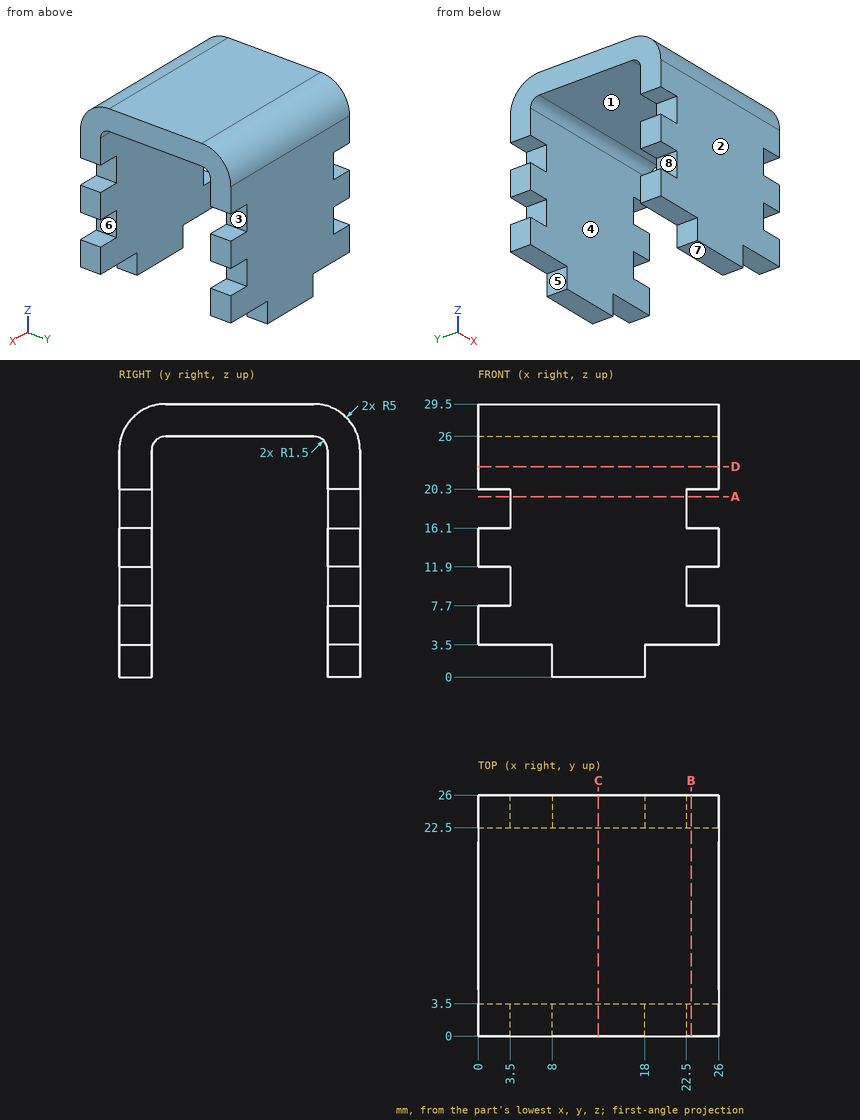
Design review of the part shown in the three views and the two pictorial views. Dimensions are in mm from the part's minimum x, y and z. A direction names the side the tool comes from. Round coordinates to 2 decimals unless told otherwise and drop trailing zeros. Write each loop counter-clockwise with the first axis right and the second up, starting at its lowest first coordinate (ties: lowest second). Pieces come first, ordered by that corner, then holes. Notation, with made-up numbers: (33.5, -5.75) -> (67.5, -5.75) arc R28 ccw to (67.5, 30.25) -> close; hole circle Ø4 at (70.5, 21). An arc over 180 degrees is marked (long way). Write item = value, one per line. Start each with the question number.
1) Take a section at B-B, the plane x = 23. State the section outline as (y, z) points, plus the area to 3 significant figures.
2) Take a section at D-D, the plane z = 22.75. State the section outline as (x, y) points.
3) Clearance check with flat-ended pins moving along their axes: pin 1 (3 mm diameter, centred on x = 1, y = 2.5, fed in from -Z); pin 2 (1 mm diameter, centred on x = 2.5, y = 1.5, fed in from +Z); pin 3 (4 mm diameter, centred on x = 23.5, y = 25, fed in from +Z). State where each tip first meets the part, or that it passes through.
4) Mouldability with a two-part tool opening along Y and no side actions: class the marked faces 1, 2 and 3 as +Y half, -Y half, draft (parallel to the pull), parting line (faces both ways), or undercut.
5) Take a section at A-A, the plane z = 19.5. State the section outline as (x, y) points.
6) Wall thickness on probe 1 along Y at (x, z) = (2, 13.25); probe 2 along Z at (x, y) = (10, 20.25); probe 3 along X at (y, z) = (22.75, 20): over which ranges is each line inside the solid? List them lowest first. Write a range as from..to.
7) Tool access review of the marked faces 4, 5, 6, 7 and 8: name each direction out of +Z, -Z, +X, -X, +Y, -Y from which nothing blocks a thin tool from reaching the whole face with its end or side.
8) Take a section at C-C, the plane x = 13. State the section outline as (y, z) points.
Results list:
q1.outline = (0, 3.5) -> (3.5, 3.5) -> (3.5, 7.7) -> (0, 7.7) -> close; (0, 11.9) -> (3.5, 11.9) -> (3.5, 16.1) -> (0, 16.1) -> close; (0, 20.3) -> (3.5, 20.3) -> (3.5, 24.5) arc R1.5 cw to (5, 26) -> (21, 26) arc R1.5 cw to (22.5, 24.5) -> (22.5, 20.3) -> (26, 20.3) -> (26, 24.5) arc R5 ccw to (21, 29.5) -> (5, 29.5) arc R5 ccw to (0, 24.5) -> close; (22.5, 3.5) -> (26, 3.5) -> (26, 7.7) -> (22.5, 7.7) -> close; (22.5, 11.9) -> (26, 11.9) -> (26, 16.1) -> (22.5, 16.1) -> close
q1.area = 180 mm²
q2.outline = (0, 0) -> (26, 0) -> (26, 3.5) -> (0, 3.5) -> close; (0, 22.5) -> (26, 22.5) -> (26, 26) -> (0, 26) -> close
q3.pin_1 = 3.5
q3.pin_2 = 28.5
q3.pin_3 = 29.08
q4.face_1 = undercut
q4.face_2 = -Y half
q4.face_3 = draft
q5.outline = (3.5, 0) -> (22.5, 0) -> (22.5, 3.5) -> (3.5, 3.5) -> close; (3.5, 22.5) -> (22.5, 22.5) -> (22.5, 26) -> (3.5, 26) -> close
q6.probe_1 = 0..3.5, 22.5..26
q6.probe_2 = 26..29.5
q6.probe_3 = 3.5..22.5
q7.face_4 = -Z, +X, -X
q7.face_5 = -Z, -X, +Y, -Y
q7.face_6 = +X, +Y, -Y
q7.face_7 = -Z, +X, -X, +Y, -Y
q7.face_8 = -X, +Y, -Y
q8.outline = (0, 0) -> (3.5, 0) -> (3.5, 24.5) arc R1.5 cw to (5, 26) -> (21, 26) arc R1.5 cw to (22.5, 24.5) -> (22.5, 0) -> (26, 0) -> (26, 24.5) arc R5 ccw to (21, 29.5) -> (5, 29.5) arc R5 ccw to (0, 24.5) -> close
